from build123d import *

# Parameters (mm, degrees)
F1_R           = 12.7
F3_R           = 2.54
F6_DEPTH       = 6.35
F6_DEPTH_BACK  = 31.75
F7_R           = 3.175
F8_DEPTH       = 40.64
F10_R          = 3.175
F11_DEPTH      = 6.35
F12_R          = 3.175
F13_DEPTH      = 19.05
F13_DEPTH_BACK = 25.4
F15_DEPTH      = 25.4
F15_DEPTH_BACK = 25.4


with BuildPart() as f2:
    # F2: sweep along a path in F0
    with BuildLine(Plane.XZ) as f2_path:
        ThreePointArc((-89.2972339832, 656.59), (-24.04175279, 594.6789825982), (0, 508))
        Line((0, 508), (0, 0))
    # F1 (on Top) → F2 (sweep)
    with BuildSketch(Plane.XY):
        Circle(F1_R)
    sweep(path=f2_path.line)

    # F3
    f3_edges = [f2.edges().sort_by_distance(p)[0] for p in [
        (-95.25782, 0, 645.37566),
        (-12.7, 0, 0),
    ]]
    fillet(f3_edges, radius=F3_R)

    # F5 (on offset) → F6 (cut, two sides)
    with BuildSketch(Plane.XZ.offset(12.7)) as f6_sk:
        with BuildLine():
            ThreePointArc((0, 479.425), (2.2450640303, 480.3549359697), (3.175, 482.6))
            ThreePointArc((3.175, 482.6), (-2.2450640303, 484.8450640303), (0, 479.425))
        make_face()
    extrude(amount=F6_DEPTH, mode=Mode.SUBTRACT)
    extrude(f6_sk.sketch, amount=-F6_DEPTH_BACK, mode=Mode.SUBTRACT)

    # F7 (on offset) → F8 (cut)
    with BuildSketch(Plane.XZ.offset(12.7)):
        with Locations((-53.642109759, 631.19)):
            Circle(F7_R)
    extrude(amount=-F8_DEPTH, mode=Mode.SUBTRACT)

    # F10 (on offset) → F11 (cut)
    with BuildSketch(Plane.XZ.offset(-12.7)):
        with Locations((-53.642109759, 631.19)):
            Circle(F10_R)
    extrude(amount=F11_DEPTH, mode=Mode.SUBTRACT)

    # F12 (on Right) → F13 (cut, two sides)
    with BuildSketch(Plane.YZ) as f13_sk:
        with Locations((0, 304.8)):
            Circle(F12_R)
        with Locations((0, 177.8)):
            Circle(F12_R)
    extrude(amount=F13_DEPTH, mode=Mode.SUBTRACT)
    extrude(f13_sk.sketch, amount=-F13_DEPTH_BACK, mode=Mode.SUBTRACT)

    # F14 (on Front) → F15 (cut, two sides)
    with BuildSketch(Plane.XZ) as f15_sk:
        with BuildLine():
            ThreePointArc((0, 9.525), (2.2450640303, 10.4549359697), (3.175, 12.7))
            ThreePointArc((3.175, 12.7), (-2.2450640303, 14.9450640303), (0, 9.525))
        make_face()
    extrude(amount=-F15_DEPTH, mode=Mode.SUBTRACT)
    extrude(f15_sk.sketch, amount=F15_DEPTH_BACK, mode=Mode.SUBTRACT)


solid = f2.part
Can you work these out from the model? Positions are in its coordinate system, mm. A direction names the side the tool comes from. Round coordinates to 2 decimals unless told otherwise and drop trailing zeros. Order: outer loops, then holes, each group sorted by start corner. A loop starts at its lowest first (then second) coordinate and runs counter-clockwise, first axis right, second up. Notation, with made-up numbers: M 16.25,-6 L 26.25,-6 A19 cw 26.25,5 Z; hole C 77.5,84.5 d9. An arc over 180 degrees is marked long. Use a Markdown table: item, result.
1) On a 3-axis mill with a long thin cutter (end or side, diameter ignored), from which of +Z, -Z, +X, -X, +Y, -Y can I reach the whole of each face in a straight line? I mean faces 1 (the face through (0, 0, 0)), 2 (the face through (12.114, -3.815, 251.732)). Say none if no direction works.
Geometry says:
| item | result |
|---|---|
| face 1 | -Z, +X, -X, +Y, -Y |
| face 2 | -Z |
2) Imagine slicing it at A-A (z = 191). List the corners of the cut face in (x, y) for me, then the cut area to 3 significant figures.
Geometry says:
| item | result |
|---|---|
| outline | C 0,0 d25.4 |
| area | 507 mm² |
3) I'm going to push flat-ended pins straight in: P1, Ø1, axis at x = -26, y = 7, coming from the +Z side; P2, Ø1, axis at x = -64, y = 7.5, coming from the +Z side; P3, Ø1.5, axis at y = 2, z = 532.5, coming from the -X side. Where does each tip first touch, or does it pass through?
Geometry says:
| item | result |
|---|---|
| P1 | stops at z = 617.25 |
| P2 | stops at z = 653.47 |
| P3 | stops at x = -14.64 |
4) If I drill on line 1 along Z through (x, y) = (-4.25, 0) (3 decimals); line 2 along X through (y, z) = (-7.5, 356.5); line 3 along Z through (x, y) = (-9.25, 0) (3 decimals), over which ranges is the centre line in solid material (lowest first)?
Geometry says:
| item | result |
|---|---|
| line 1 | z = 0 to 174.625, 180.975 to 301.625, 307.975 to 584.471 |
| line 2 | x = -10.25 to 10.25 |
| line 3 | z = 0 to 174.625, 180.975 to 301.625, 307.975 to 594.389 |
